```python
from build123d import *

# Parameters (mm, degrees)
F0_R     = 10.7
F1_DEPTH = 3.5
F0_R_2   = 10.2
F2_DEPTH = 1.25


with BuildPart() as f1:
    # F0 (on Top) → F1 (new body)
    with BuildSketch(Plane.XY):
        with BuildLine():
            Line((-15.105254, 24.721022), (-7.114419, 10.880489))
            ThreePointArc((-7.114419, 10.880489), (-5.017235, 11.992804), (-2.752749, 12.70521))
            Line((-2.752749, 12.70521), (-6.445, 14.836933))
            Line((-6.445, 14.836933), (-6.445, 22.278978))
            Line((-6.445, 22.278978), (-12.89, 26))
            Line((-12.89, 26), (-12.89, 33.442045))
            Line((-12.89, 33.442045), (-6.445, 37.163067))
            Line((-6.445, 37.163067), (0, 33.442045))
            Line((0, 33.442045), (6.445, 37.163067))
            Line((6.445, 37.163067), (12.89, 33.442045))
            Line((12.89, 33.442045), (12.89, 26))
            Line((12.89, 26), (6.445, 22.278978))
            Line((6.445, 22.278978), (6.445, 14.836933))
            Line((6.445, 14.836933), (2.752749, 12.70521))
            ThreePointArc((2.752749, 12.70521), (5.017235, 11.992804), (7.114419, 10.880489))
            Line((7.114419, 10.880489), (15.105254, 24.721022))
            ThreePointArc((15.105254, 24.721022), (12.864302, 37.388653), (0, 37.367066))
            ThreePointArc((0, 37.367066), (-12.864302, 37.388653), (-15.105254, 24.721022))
        make_face()
        with BuildLine():
            ThreePointArc((-12.979989, 0.721022), (-12.894691, -1.651349), (-12.37941, -3.968655))
            Line((-12.37941, -3.968655), (-9.62666, -5.557955))
            Line((-9.62666, -5.557955), (-9.62666, -8.736556))
            ThreePointArc((-9.62666, -8.736556), (-7.877455, -10.341455), (-5.865571, -11.601512))
            ThreePointArc((-5.865571, -11.601512), (0, -13), (5.865571, -11.601512))
            ThreePointArc((5.865571, -11.601512), (7.877455, -10.341455), (9.62666, -8.736556))
            Line((9.62666, -8.736556), (9.62666, -5.557955))
            Line((9.62666, -5.557955), (12.37941, -3.968655))
            ThreePointArc((12.37941, -3.968655), (12.894691, -1.651349), (12.979989, 0.721022))
            ThreePointArc((12.979989, 0.721022), (11.25833, 6.5), (7.114419, 10.880489))
            ThreePointArc((7.114419, 10.880489), (5.017235, 11.992804), (2.752749, 12.70521))
            Line((2.752749, 12.70521), (0, 11.11591))
            Line((0, 11.11591), (-2.752749, 12.70521))
            ThreePointArc((-2.752749, 12.70521), (-5.017235, 11.992804), (-7.114419, 10.880489))
            ThreePointArc((-7.114419, 10.880489), (-11.25833, 6.5), (-12.979989, 0.721022))
        make_face()
        Circle(F0_R, mode=Mode.SUBTRACT)
        with BuildLine():
            ThreePointArc((9.62666, -8.736556), (7.877455, -10.341455), (5.865571, -11.601512))
            Line((5.865571, -11.601512), (13.856406, -25.442045))
            ThreePointArc((13.856406, -25.442045), (25.947372, -29.835139), (32.360828, -18.683533))
            ThreePointArc((32.360828, -18.683533), (38.811675, -7.553514), (28.96166, 0.721022))
            Line((28.96166, 0.721022), (12.979989, 0.721022))
            ThreePointArc((12.979989, 0.721022), (12.894691, -1.651349), (12.37941, -3.968655))
            Line((12.37941, -3.968655), (16.07166, -1.836933))
            Line((16.07166, -1.836933), (22.51666, -5.557955))
            Line((22.51666, -5.557955), (28.96166, -1.836933))
            Line((28.96166, -1.836933), (35.40666, -5.557955))
            Line((35.40666, -5.557955), (35.40666, -13))
            Line((35.40666, -13), (28.96166, -16.721022))
            Line((28.96166, -16.721022), (28.96166, -24.163067))
            Line((28.96166, -24.163067), (22.51666, -27.88409))
            Line((22.51666, -27.88409), (16.07166, -24.163067))
            Line((16.07166, -24.163067), (16.07166, -16.721022))
            Line((16.07166, -16.721022), (9.62666, -13))
            Line((9.62666, -13), (9.62666, -8.736556))
        make_face()
        with BuildLine():
            Line((-28.96166, -24.163067), (-28.96166, -16.721022))
            Line((-28.96166, -16.721022), (-35.40666, -13))
            Line((-35.40666, -13), (-35.40666, -5.557955))
            Line((-35.40666, -5.557955), (-28.96166, -1.836933))
            Line((-28.96166, -1.836933), (-22.51666, -5.557955))
            Line((-22.51666, -5.557955), (-16.07166, -1.836933))
            Line((-16.07166, -1.836933), (-12.37941, -3.968655))
            ThreePointArc((-12.37941, -3.968655), (-12.894691, -1.651349), (-12.979989, 0.721022))
            Line((-12.979989, 0.721022), (-28.96166, 0.721022))
            ThreePointArc((-28.96166, 0.721022), (-38.811675, -7.553514), (-32.360828, -18.683533))
            ThreePointArc((-32.360828, -18.683533), (-25.947372, -29.835139), (-13.856406, -25.442045))
            Line((-13.856406, -25.442045), (-5.865571, -11.601512))
            ThreePointArc((-5.865571, -11.601512), (-7.877455, -10.341455), (-9.62666, -8.736556))
            Line((-9.62666, -8.736556), (-9.62666, -13))
            Line((-9.62666, -13), (-16.07166, -16.721022))
            Line((-16.07166, -16.721022), (-16.07166, -24.163067))
            Line((-16.07166, -24.163067), (-22.51666, -27.88409))
            Line((-22.51666, -27.88409), (-28.96166, -24.163067))
        make_face()
    extrude(amount=F1_DEPTH)

    # F0 (on Top) → F2 (join)
    with BuildSketch(Plane.XY):
        with BuildLine():
            Line((-28.96166, -24.163067), (-28.96166, -16.721022))
            Line((-28.96166, -16.721022), (-35.40666, -13))
            Line((-35.40666, -13), (-35.40666, -5.557955))
            Line((-35.40666, -5.557955), (-28.96166, -1.836933))
            Line((-28.96166, -1.836933), (-22.51666, -5.557955))
            Line((-22.51666, -5.557955), (-16.07166, -1.836933))
            Line((-16.07166, -1.836933), (-12.37941, -3.968655))
            ThreePointArc((-12.37941, -3.968655), (-12.894691, -1.651349), (-12.979989, 0.721022))
            Line((-12.979989, 0.721022), (-28.96166, 0.721022))
            ThreePointArc((-28.96166, 0.721022), (-38.811675, -7.553514), (-32.360828, -18.683533))
            ThreePointArc((-32.360828, -18.683533), (-25.947372, -29.835139), (-13.856406, -25.442045))
            Line((-13.856406, -25.442045), (-5.865571, -11.601512))
            ThreePointArc((-5.865571, -11.601512), (-7.877455, -10.341455), (-9.62666, -8.736556))
            Line((-9.62666, -8.736556), (-9.62666, -13))
            Line((-9.62666, -13), (-16.07166, -16.721022))
            Line((-16.07166, -16.721022), (-16.07166, -24.163067))
            Line((-16.07166, -24.163067), (-22.51666, -27.88409))
            Line((-22.51666, -27.88409), (-28.96166, -24.163067))
        make_face()
        with BuildLine():
            ThreePointArc((-12.979989, 0.721022), (-12.894691, -1.651349), (-12.37941, -3.968655))
            Line((-12.37941, -3.968655), (-9.62666, -5.557955))
            Line((-9.62666, -5.557955), (-9.62666, -8.736556))
            ThreePointArc((-9.62666, -8.736556), (-7.877455, -10.341455), (-5.865571, -11.601512))
            ThreePointArc((-5.865571, -11.601512), (0, -13), (5.865571, -11.601512))
            ThreePointArc((5.865571, -11.601512), (7.877455, -10.341455), (9.62666, -8.736556))
            Line((9.62666, -8.736556), (9.62666, -5.557955))
            Line((9.62666, -5.557955), (12.37941, -3.968655))
            ThreePointArc((12.37941, -3.968655), (12.894691, -1.651349), (12.979989, 0.721022))
            ThreePointArc((12.979989, 0.721022), (11.25833, 6.5), (7.114419, 10.880489))
            ThreePointArc((7.114419, 10.880489), (5.017235, 11.992804), (2.752749, 12.70521))
            Line((2.752749, 12.70521), (0, 11.11591))
            Line((0, 11.11591), (-2.752749, 12.70521))
            ThreePointArc((-2.752749, 12.70521), (-5.017235, 11.992804), (-7.114419, 10.880489))
            ThreePointArc((-7.114419, 10.880489), (-11.25833, 6.5), (-12.979989, 0.721022))
        make_face()
        Circle(F0_R, mode=Mode.SUBTRACT)
        with BuildLine():
            Line((-15.105254, 24.721022), (-7.114419, 10.880489))
            ThreePointArc((-7.114419, 10.880489), (-5.017235, 11.992804), (-2.752749, 12.70521))
            Line((-2.752749, 12.70521), (-6.445, 14.836933))
            Line((-6.445, 14.836933), (-6.445, 22.278978))
            Line((-6.445, 22.278978), (-12.89, 26))
            Line((-12.89, 26), (-12.89, 33.442045))
            Line((-12.89, 33.442045), (-6.445, 37.163067))
            Line((-6.445, 37.163067), (0, 33.442045))
            Line((0, 33.442045), (6.445, 37.163067))
            Line((6.445, 37.163067), (12.89, 33.442045))
            Line((12.89, 33.442045), (12.89, 26))
            Line((12.89, 26), (6.445, 22.278978))
            Line((6.445, 22.278978), (6.445, 14.836933))
            Line((6.445, 14.836933), (2.752749, 12.70521))
            ThreePointArc((2.752749, 12.70521), (5.017235, 11.992804), (7.114419, 10.880489))
            Line((7.114419, 10.880489), (15.105254, 24.721022))
            ThreePointArc((15.105254, 24.721022), (12.864302, 37.388653), (0, 37.367066))
            ThreePointArc((0, 37.367066), (-12.864302, 37.388653), (-15.105254, 24.721022))
        make_face()
        with BuildLine():
            ThreePointArc((9.62666, -8.736556), (7.877455, -10.341455), (5.865571, -11.601512))
            Line((5.865571, -11.601512), (13.856406, -25.442045))
            ThreePointArc((13.856406, -25.442045), (25.947372, -29.835139), (32.360828, -18.683533))
            ThreePointArc((32.360828, -18.683533), (38.811675, -7.553514), (28.96166, 0.721022))
            Line((28.96166, 0.721022), (12.979989, 0.721022))
            ThreePointArc((12.979989, 0.721022), (12.894691, -1.651349), (12.37941, -3.968655))
            Line((12.37941, -3.968655), (16.07166, -1.836933))
            Line((16.07166, -1.836933), (22.51666, -5.557955))
            Line((22.51666, -5.557955), (28.96166, -1.836933))
            Line((28.96166, -1.836933), (35.40666, -5.557955))
            Line((35.40666, -5.557955), (35.40666, -13))
            Line((35.40666, -13), (28.96166, -16.721022))
            Line((28.96166, -16.721022), (28.96166, -24.163067))
            Line((28.96166, -24.163067), (22.51666, -27.88409))
            Line((22.51666, -27.88409), (16.07166, -24.163067))
            Line((16.07166, -24.163067), (16.07166, -16.721022))
            Line((16.07166, -16.721022), (9.62666, -13))
            Line((9.62666, -13), (9.62666, -8.736556))
        make_face()
        Polygon((22.51666, -13), (16.07166, -16.721022), (16.07166, -24.163067), (22.51666, -27.88409), (28.96166, -24.163067), (28.96166, -16.721022), align=None)
        Polygon((0, 33.442045), (0, 26), (6.445, 22.278978), (12.89, 26), (12.89, 33.442045), (6.445, 37.163067), align=None)
        Polygon((-12.89, 26), (-6.445, 22.278978), (0, 26), (0, 33.442045), (-6.445, 37.163067), (-12.89, 33.442045), align=None)
        Polygon((-6.445, 14.836933), (-2.752749, 12.70521), (0, 11.11591), (2.752749, 12.70521), (6.445, 14.836933), (6.445, 22.278978), (0, 26), (-6.445, 22.278978), align=None)
        Polygon((22.51666, -5.557955), (22.51666, -13), (28.96166, -16.721022), (35.40666, -13), (35.40666, -5.557955), (28.96166, -1.836933), align=None)
        Polygon((9.62666, -5.557955), (9.62666, -8.736556), (9.62666, -13), (16.07166, -16.721022), (22.51666, -13), (22.51666, -5.557955), (16.07166, -1.836933), (12.37941, -3.968655), align=None)
        Polygon((-22.51666, -5.557955), (-22.51666, -13), (-16.07166, -16.721022), (-9.62666, -13), (-9.62666, -8.736556), (-9.62666, -5.557955), (-12.37941, -3.968655), (-16.07166, -1.836933), align=None)
        Polygon((-28.96166, -16.721022), (-22.51666, -13), (-22.51666, -5.557955), (-28.96166, -1.836933), (-35.40666, -5.557955), (-35.40666, -13), align=None)
        Polygon((-16.07166, -16.721022), (-22.51666, -13), (-28.96166, -16.721022), (-28.96166, -24.163067), (-22.51666, -27.88409), (-16.07166, -24.163067), align=None)
        Circle(F0_R)
        Circle(F0_R_2, mode=Mode.SUBTRACT)
    extrude(amount=-F2_DEPTH)


solid = f1.part
```
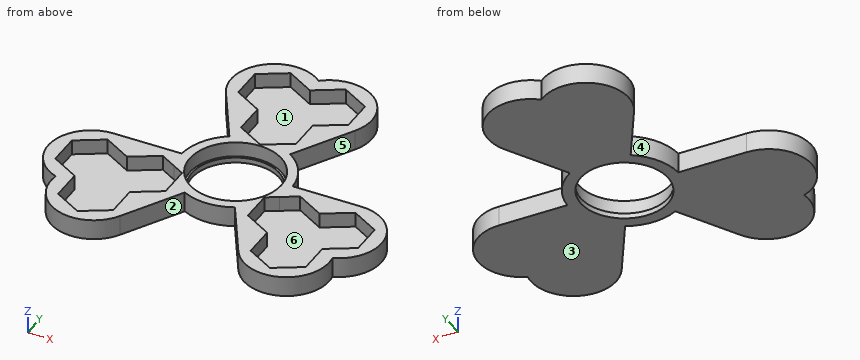
Geometry: final body of the model. Coordinates: model frame, mm. Face numbers are marked on the shaded views. A direction names the side the tool comes from. Round coordinates to 2 decimals unless told otherwise and drop trailing zeros. Write each loop counter-clockwise with the first axis right and the second up, starting at its lowest first coordinate (ties: lowest second). Pieces come first, ordered by that corner, then holes. Notation, with made-up numbers: M 42.25,-3 L 59.25,-3 A15 ccw 59.25,23 Z; hole C 69,75 d4. An arc over 180 degrees is marked long. Answer in a Markdown table with one row per item. Add a question column.
(1) Contact query for flat-ended pins moving along their axis: pin 1 (1 mm diameter, centred on y = -22, z = 1.5, fed in from -X); pin 2 (6.5 mm diameter, centred on x = 4, y = 4, fed in from +Z); pin 3 (2 mm diameter, centred on y = -14.5, z = 1, fed in from +X); pin 4 (1.4 mm diameter, centred on x = -19, z = 2, fed in from +Y). Output: stop coordinate, or through.
(2) Ray query, L1, parallel to Y at x = 12, z = 0.3; L2, parallel to Y at x = -9, z = 1.55; L3, parallel to Z at x = 12, y = 31. Return the intervals inside material, ascending.
(3) Draft query along Y for the marked faces 1, 2 and 3. Return one class per face: pulls with the +Y half, pulls with the -Y half, needs draft (parallel to the pull), parting line crosses it, or undercut.
(4) Cut plane B-B, the plane x = -27.5. Return the cut outline in (y, z).
(5) Cut plane C-C, the plane z = 2.3. Give the number of separate pieces and of enclosed holes in the cut face, then the cut area to 3 significant figures.
(6) Reachability of the marked faces 4, 5 and 6 from +Z, -Z, +X, -X, +Y, -Y: full face, straight path, thin tool, end or side. Return the list, or none.
(7) Cut plane A-A, the plane y = -20. Return the cut outline in (x, z), then the cut area to 3 significant figures.
Established:
| question | item | result |
|---|---|---|
| 1 | pin 1 | x = -32.46 |
| 1 | pin 2 | through |
| 1 | pin 3 | x = 38.03 |
| 1 | pin 4 | y = 0.72 |
| 2 | L1 | -22.23 to -14.37, -4.19 to 5, 19.34 to 25.49, 33.96 to 38.04 |
| 2 | L2 | -17.03 to -5.79, 5.79 to 9.38, 14.15 to 23.75, 35.69 to 39.39 |
| 2 | L3 | -1.25 to 0 |
| 3 | face 1 | undercut |
| 3 | face 2 | pulls with the -Y half |
| 3 | face 3 | needs draft |
| 4 | outline | M -29.11,-1.25 L 0.72,-1.25 L 0.72,3.5 L -2.68,3.5 L -2.68,0 L -25.01,0 L -25.01,3.5 L -29.11,3.5 Z |
| 5 | separate pieces | 1 |
| 5 | enclosed holes | 4 |
| 5 | area | 1,050 mm² |
| 6 | face 4 | +Z, -Z, -X |
| 6 | face 5 | +Z, -Z, +X |
| 6 | face 6 | +Z |
| 7 | outline | M -32.51,-1.25 L -10.71,-1.25 L -10.71,3.5 L -16.07,3.5 L -16.07,0 L -28.96,0 L -28.96,3.5 L -32.51,3.5 Z; M 10.71,-1.25 L 32.51,-1.25 L 32.51,3.5 L 28.96,3.5 L 28.96,0 L 16.07,0 L 16.07,3.5 L 10.71,3.5 Z |
| 7 | area | 117 mm² |
